Can you work these out from the model? Positions are in its coordinate system, mm. Face numbers are marked on the shaded views. Round coordinates to 2 decimals unless told otherwise and drop trailing zeros. Loops run counter-clockwise (first coordinate to the right, second up) from the corner with the lowest first, then second, coordinate; pieces in that order, holes last.
(1) I want a section at D-D on y = -11.5. Write out the boundary of the cut face in (x, z), plus the area to 3 significant figures.
(2) If I drill on line 1 along Y through (x, z) = (17.5, 0.5); line 2 along Y through (x, z) = (-3.5, 3); line 3 along X through (y, z) = (4.5, 7.25), over which ranges is the centre line in solid material (lowest first)?
(3) I want a section at A-A on y = 4. Write out the boundary of the cut face in (x, z).
(4) Thinking about a two-plate mould opening in Y: for the marked faces 1, 2 and 3, which applies, released by +Y, released by -Y, zero draft, split by the parting line, or undercut?
(5) I want a section at B-B on x = -1.5. Write out the boundary of the cut face in (y, z), plus the area to 3 significant figures.
(6) I want a section at C-C on z = 3. Write out the boundary of the cut face in (x, y), plus the area to 3 significant figures.
Autodesk Inventor part; units mm, degrees
ref_plane "YZ Plane" through (0, 0, 0) normal (1, 0, 0) x (0, 1, 0)
ref_plane "XZ Plane" through (0, 0, 0) normal (0, 1, 0) x (-1, 0, 0)
ref_plane "XY Plane" through (0, 0, 0) normal (0, 0, 1) x (1, 0, 0)
sketch "Sketch1" plane through (0, 0, 0) normal (0, 0, 1) x (1, 0, 0)
  line L0 (-13.9136, 8.9772) -> (28.0864, 8.9772)
  line L1 (28.0864, 8.9772) -> (28.0864, -13.0228)
  line L2 (28.0864, -13.0228) -> (-13.9136, -13.0228)
  line L3 (-13.9136, -13.0228) -> (-13.9136, 8.9772)
  point P0 (0, 0)
  dimension "d0" = 42
  dimension "d1" = 22
extrude "Extrusion1" add sketch "Sketch1" along normal blind 10
sketch "Sketch2" plane through (0, 0, 10) normal (0, 0, 1) x (1, 0, 0)
  line L0 (-13.9136, -13.0228) -> (28.0864, -13.0228)
  arc A0 (-3.4134, -5.6894) -> (-3.4136, -13.0228) centre (-3.4136, -9.3561) ccw
  arc A1 (-3.4134, -5.6894) -> (-3.4134, 1.6439) centre (-3.4133, -2.0228) ccw
  arc A2 (17.5864, -13.0228) -> (17.5862, -5.6894) centre (17.5864, -9.3561) ccw
  arc A3 (17.5862, 1.6439) -> (17.5862, -5.6894) centre (17.586, -2.0228) ccw
  line L1 (-3.4136, -13.0228) -> (17.5864, -13.0228)
  line L2 (-3.4135, 8.9772) -> (17.5865, 8.9772)
  line L3 (28.0864, 8.9772) -> (-13.9136, 8.9772)
  line L4 (-3.4133, -2.0228) -> (-3.4136, -9.3561) construction
  line L5 (17.5864, -9.3561) -> (17.586, -2.0228) construction
  arc A4 (-3.4135, 8.9772) -> (-3.4134, 1.6439) centre (-3.4136, 5.3106) ccw
  arc A5 (17.5862, 1.6439) -> (17.5865, 8.9772) centre (17.5864, 5.3106) ccw
  line L6 (-3.4133, -2.0228) -> (-13.9136, -2.0228) construction
  line L7 (17.586, -2.0228) -> (28.0864, -2.0228) construction
  line L8 (28.0864, -13.0228) -> (28.0864, 8.9772) construction
  line L9 (-13.9136, 8.9772) -> (-13.9136, -13.0228)
  line L10 (-7.0803, -9.356) -> (-13.9136, -9.356) construction
  line L11 (21.2531, -9.356) -> (28.0864, -9.356) construction
  line L12 (-13.9136, -13.0228) -> (28.0864, -13.0228)
  line L13 (28.0864, -13.0228) -> (28.0864, 8.9772)
  line L14 (28.0864, 8.9772) -> (-13.9136, 8.9772)
  line L15 (-13.9136, 8.9772) -> (-13.9136, -13.0228)
  line L16 (-7.0803, 5.3105) -> (-13.9136, 5.3105) construction
  line L17 (21.2531, 5.3105) -> (28.0864, 5.3105) construction
  point P0 (0, 0)
  point P1 (17.8152, 8.9772)
  point P2 (-3.4136, 8.9772)
  point P3 (-3.4136, 8.9772)
  dimension "d4" = 21
  dimension "d5" = 22
  dimension "d17" = 21
extrude "Extrusion2" cut sketch "Sketch2" against normal blind 10 contours L9 L3 A4 A1 A0 L0 | A2 A3 A5 L3 L13 L0
sketch "Sketch3" plane through (0, 0, 10) normal (0, 0, 1) x (1, 0, 0)
  arc A0 (-3.4134, -5.6894) -> (-3.4134, 1.6439) centre (-3.4133, -2.0228) ccw construction
  line L0 (-7.2207, -5.6893) -> (3.1864, -5.6897) construction
  line L1 (20.3968, -5.6893) -> (9.686, -5.6898) construction
  arc A1 (-3.4134, -5.6894) -> (-3.4136, -13.0228) centre (-3.4136, -9.3561) ccw construction
  arc A2 (-3.4134, -5.6894) -> (-3.4134, 1.6439) centre (-3.4133, -2.0228) ccw construction
  arc A3 (17.5864, -13.0228) -> (17.5862, -5.6894) centre (17.5864, -9.3561) ccw construction
  arc A4 (17.5862, 1.6439) -> (17.5862, -5.6894) centre (17.586, -2.0228) ccw construction
  line L2 (-3.4137, -11.3763) -> (-3.4129, 5.1845) construction
  line L3 (17.5866, -13.0364) -> (17.5857, 5.1238) construction
  arc A5 (17.5862, 1.6439) -> (17.5862, -5.6894) centre (17.586, -2.0228) ccw construction
  point P0 (0, 0)
hole "Hole1" at (-3.4129, 5.1845, 10) at (17.5857, 5.1238, 10) direction (0, 0, -1) diameter 3 end through all
properties part number "Zipperteethv6"
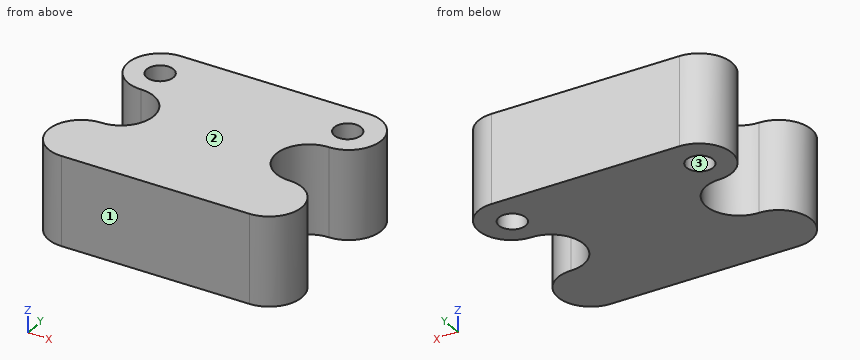
Filled sheet:
1. outline: (-6.39, 0) - (20.56, 0) - (20.56, 10) - (-6.39, 10) - close
1. area: 269 mm2
2. line 1: y = -13.02 to -5.69, 1.64 to 3.63, 6.62 to 8.98
2. line 2: y = -13.02 to -5.69, 1.64 to 3.69, 6.68 to 8.98
2. line 3: x = -6.99 to -4.75, -2.08 to 16.22, 18.95 to 21.16
3. outline: (-6.84, 0) - (-4.33, 0) - (-4.33, 10) - (-6.84, 10) - close; (-2.49, 0) - (16.59, 0) - (16.59, 10) - (-2.49, 10) - close; (18.58, 0) - (21.01, 0) - (21.01, 10) - (18.58, 10) - close
4. face 1: released by -Y
4. face 2: zero draft
4. face 3: undercut
5. outline: (-13.02, 0) - (-5.15, 0) - (-5.15, 10) - (-13.02, 10) - close; (1.11, 0) - (8.98, 0) - (8.98, 10) - (1.11, 10) - close
5. area: 157 mm2
6. outline: (-3.41, -13.02) - (17.59, -13.02) arc R3.67 ccw to (17.59, -5.69) arc R3.67 cw to (17.59, 1.64) arc R3.67 ccw to (17.59, 8.98) - (-3.41, 8.98) arc R3.67 ccw to (-3.41, 1.64) arc R3.67 cw to (-3.41, -5.69) arc R3.67 ccw to start; hole circle Ø3 at (-3.41, 5.18); hole circle Ø3 at (17.59, 5.12)
6. area: 490 mm2
